from build123d import *

# Parameters (mm, degrees)
SKETCH1_R             = 26
BOSS_EXTRUDE1_DEPTH   = 15
BOSS_EXTRUDE2_DEPTH   = 15
CHAMFER1_SIZE         = 2
CHAMFER1_SIZE2        = 0.727940469
CHAMFER1_PART_2_SIZE  = 2
CHAMFER1_PART_2_SIZE2 = 0.727940469
CHAMFER1_PART_3_SIZE  = 2
CHAMFER1_PART_3_SIZE2 = 0.727940469
CHAMFER1_PART_4_SIZE  = 2
CHAMFER1_PART_4_SIZE2 = 0.727940469
CHAMFER1_PART_5_SIZE  = 2
CHAMFER1_PART_5_SIZE2 = 0.727940469
CHAMFER1_PART_6_SIZE  = 2
CHAMFER1_PART_6_SIZE2 = 0.727940469
CHAMFER2_SIZE         = 2
CHAMFER2_SIZE2        = 0.727940469
SKETCH3_R             = 3.25
CUT_EXTRUDE1_DEPTH    = 18
CHAMFER3_SIZE         = 1


with BuildPart() as part:
    # Sketch1 → Boss-Extrude1 (new body, symmetric)
    with BuildSketch(Plane(origin=(0, 0, 0), x_dir=(1, 0, 0), z_dir=(0, 1, 0))):
        Circle(SKETCH1_R)
    extrude(amount=BOSS_EXTRUDE1_DEPTH, both=True)

    # Sketch2 → Boss-Extrude2 (add)
    with BuildSketch(Plane(origin=(0, 15, 0), x_dir=(1, 0, 0), z_dir=(0, 1, 0))):
        Polygon((-17.320508076, 0), (-8.660254038, -15), (8.660254038, -15), (17.320508076, 0), (8.660254038, 15), (-8.660254038, 15), align=None)
    extrude(amount=BOSS_EXTRUDE2_DEPTH)

    # Chamfer1
    chamfer1_edges = [part.edges().sort_by_distance(p)[0] for p in [
        (-12.990381057, 30, -7.5),
    ]]
    chamfer1_side = [part.faces().sort_by_distance(p)[0] for p in [
        (-12.990381057, 22.5, -7.5),
    ]]
    chamfer(chamfer1_edges, length=CHAMFER1_SIZE, length2=CHAMFER1_SIZE2, reference=chamfer1_side[0])

    # Chamfer1 part 2
    chamfer1_part_2_edges = [part.edges().sort_by_distance(p)[0] for p in [
        (-12.990381057, 30, 7.5),
    ]]
    chamfer1_part_2_side = [part.faces().sort_by_distance(p)[0] for p in [
        (-12.990381057, 22.5, 7.5),
    ]]
    chamfer(chamfer1_part_2_edges, length=CHAMFER1_PART_2_SIZE, length2=CHAMFER1_PART_2_SIZE2, reference=chamfer1_part_2_side[0])

    # Chamfer1 part 3
    chamfer1_part_3_edges = [part.edges().sort_by_distance(p)[0] for p in [
        (0, 30, 15),
    ]]
    chamfer1_part_3_side = [part.faces().sort_by_distance(p)[0] for p in [
        (0, 22.5, 15),
    ]]
    chamfer(chamfer1_part_3_edges, length=CHAMFER1_PART_3_SIZE, length2=CHAMFER1_PART_3_SIZE2, reference=chamfer1_part_3_side[0])

    # Chamfer1 part 4
    chamfer1_part_4_edges = [part.edges().sort_by_distance(p)[0] for p in [
        (12.990381057, 30, 7.5),
    ]]
    chamfer1_part_4_side = [part.faces().sort_by_distance(p)[0] for p in [
        (12.990381057, 22.5, 7.5),
    ]]
    chamfer(chamfer1_part_4_edges, length=CHAMFER1_PART_4_SIZE, length2=CHAMFER1_PART_4_SIZE2, reference=chamfer1_part_4_side[0])

    # Chamfer1 part 5
    chamfer1_part_5_edges = [part.edges().sort_by_distance(p)[0] for p in [
        (12.990381057, 30, -7.5),
    ]]
    chamfer1_part_5_side = [part.faces().sort_by_distance(p)[0] for p in [
        (12.990381057, 22.5, -7.5),
    ]]
    chamfer(chamfer1_part_5_edges, length=CHAMFER1_PART_5_SIZE, length2=CHAMFER1_PART_5_SIZE2, reference=chamfer1_part_5_side[0])

    # Chamfer1 part 6
    chamfer1_part_6_edges = [part.edges().sort_by_distance(p)[0] for p in [
        (0, 30, -15),
    ]]
    chamfer1_part_6_side = [part.faces().sort_by_distance(p)[0] for p in [
        (0, 22.5, -15),
    ]]
    chamfer(chamfer1_part_6_edges, length=CHAMFER1_PART_6_SIZE, length2=CHAMFER1_PART_6_SIZE2, reference=chamfer1_part_6_side[0])

    # Chamfer2
    chamfer2_edges = [part.edges().sort_by_distance(p)[0] for p in [
        (-26, -15, 0),
    ]]
    chamfer2_side = [part.faces().sort_by_distance(p)[0] for p in [
        (-26, 0, 0),
    ]]
    chamfer(chamfer2_edges, length=CHAMFER2_SIZE, length2=CHAMFER2_SIZE2, reference=chamfer2_side[0])

    # Sketch3 → Cut-Extrude1 (cut)
    with BuildSketch(Plane(origin=(0, 30, 0), x_dir=(1, 0, 0), z_dir=(0, 1, 0))):
        Circle(SKETCH3_R)
    extrude(amount=-CUT_EXTRUDE1_DEPTH, mode=Mode.SUBTRACT)

    # Chamfer3
    chamfer3_edges = [part.edges().sort_by_distance(p)[0] for p in [
        (-3.25, 30, 0),
    ]]
    chamfer(chamfer3_edges, length=CHAMFER3_SIZE)


solid = part.part
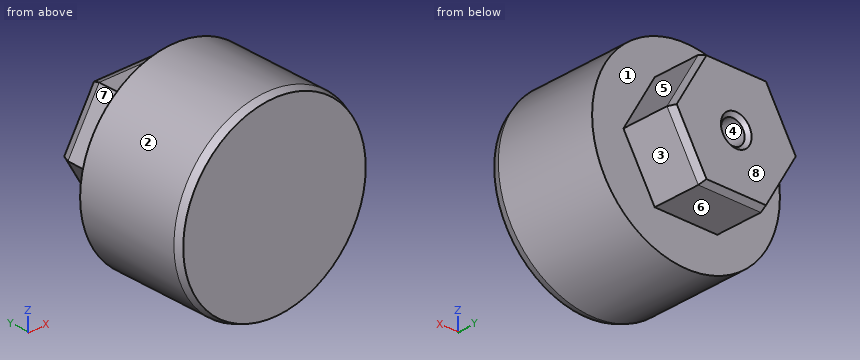
Part model, mm, in its own coordinate system. Face numbers are marked on the shaded views. A direction names the side the tool comes from. Give positions to 0.01 mm unless a question says otherwise; leave off trailing zeros. Loops run counter-clockwise (first coordinate to the right, second up) from the corner with the lowest first, then second, coordinate; pieces in that order, holes last.
(1) Drill centre lines: line 1 along X through (y, z) = (23, 0); line 2 along Y through (x, z) = (-5, 16); line 3 along Z through (x, y) = (0, 15.5). Where is each one in solid material? Low to high.
Return value:
line 1: x = -17.32 to -3.25, 3.25 to 17.32
line 2: y = -15 to 15
line 3: z = -15 to -3.25, 3.25 to 15
(2) Pin check, flat tips, straight feed: pin 1 (1.5 mm diameter, centred on y = -10, z = -7, fed in from -X); pin 2 (8 mm diameter, centred on y = 21, z = -4.5, fed in from -X); pin 3 (2 mm diameter, centred on x = 19, z = 1, fed in from +Y). Stop position of each tip, or through.
Return value:
pin 1: stops at x = -25.24
pin 2: stops at x = -17.03
pin 3: stops at y = 15
(3) 3-axis set-ups, long thin cutter, end or side, ignore diameter. For the marked faces 5, 6, 7 and 8: which of +Z, -Z, +X, -X, +Y, -Y reach the whole face in a straight line?
Return value:
face 5: +Z, +X, +Y
face 6: -Z, +X, -X, +Y
face 7: +Z, -X, +Y
face 8: +Z, -Z, +X, -X, +Y
(4) Band-saw the part on B-B (x = 0). Write the cut outline in (y, z).
Return value:
outline: (-15, -25.27) - (-13, -26) - (15, -26) - (15, -15) - (28, -15) - (30, -14.27) - (30, -4.25) - (29, -3.25) - (12, -3.25) - (12, 3.25) - (29, 3.25) - (30, 4.25) - (30, 14.27) - (28, 15) - (15, 15) - (15, 26) - (-13, 26) - (-15, 25.27) - close
(5) Band-saw the part on C-C (y = 9). Write the cut outline in (x, z).
Return value:
outline: circle Ø52 at (0, 0)
(6) Pull direction X, two halves, no side cores. Call the marked faces 1, 2, 3 and 4: pulls with the +X half, pulls with the -X half, needs draft (parallel to the pull), parting line crosses it, or undercut.
Return value:
face 1: needs draft
face 2: parting line crosses it
face 3: pulls with the +X half
face 4: undercut
(7) Band-saw the part on A-A (y = 24). Write the cut outline in (x, z), and give its area (3 significant figures).
Return value:
outline: (-17.32, 0) - (-8.66, -15) - (8.66, -15) - (17.32, 0) - (8.66, 15) - (-8.66, 15) - close; hole circle Ø6.5 at (0, 0)
area: 746 mm2
